from build123d import *

# Parameters (mm, degrees)
BOSS_EXTRUDE1_DEPTH          = 2.65684
CUT_EXTRUDE1_DEPTH           = 3.65684
SKETCH3_R                    = 16.891
CUT_EXTRUDE2_DEPTH           = 3.65684
F_10_0_1935_DIAMETER_HOLE1_D = 4.9149


with BuildPart() as part:
    # Sketch1 → Boss-Extrude1 (new body)
    with BuildSketch(Plane(origin=(0, 0, 0), x_dir=(1, 0, 0), z_dir=(0, 1, 0))):
        Polygon((-711.2, 203.2), (-711.2, 0), (711.2, 0), (711.2, 203.2), (330.2, 812.8), (-330.2, 812.8), align=None)
    extrude(amount=BOSS_EXTRUDE1_DEPTH)

    # Sketch2 → Cut-Extrude1 (cut, through all)
    with BuildSketch(Plane(origin=(0, 2.65684, 0), x_dir=(1, 0, 0), z_dir=(0, 1, 0))):
        with BuildLine():
            Line((-63.5, 781.05), (63.5, 781.05))
            ThreePointArc((63.5, 781.05), (79.375, 765.175), (63.5, 749.3))
            Line((63.5, 749.3), (-63.5, 749.3))
            ThreePointArc((-63.5, 749.3), (-79.375, 765.175), (-63.5, 781.05))
        make_face()
        with BuildLine():
            Line((-647.7, 63.5), (-520.7, 63.5))
            ThreePointArc((-520.7, 63.5), (-504.825, 47.625), (-520.7, 31.75))
            Line((-520.7, 31.75), (-647.7, 31.75))
            ThreePointArc((-647.7, 31.75), (-663.575, 47.625), (-647.7, 63.5))
        make_face()
        with BuildLine():
            Line((520.7, 63.5), (647.7, 63.5))
            ThreePointArc((647.7, 63.5), (663.575, 47.625), (647.7, 31.75))
            Line((647.7, 31.75), (520.7, 31.75))
            ThreePointArc((520.7, 31.75), (504.825, 47.625), (520.7, 63.5))
        make_face()
    extrude(amount=-CUT_EXTRUDE1_DEPTH, mode=Mode.SUBTRACT)

    # Sketch3 → Cut-Extrude2 (cut, through all)
    with BuildSketch(Plane(origin=(0, 2.65684, 0), x_dir=(1, 0, 0), z_dir=(0, 1, 0))):
        with Locations((-469.9, 224.282)):
            Circle(SKETCH3_R)
        with Locations((-225.425, 669.586361505)):
            Circle(SKETCH3_R)
        with Locations((225.425, 669.586361505)):
            Circle(SKETCH3_R)
        with Locations((469.9, 224.282)):
            Circle(SKETCH3_R)
    extrude(amount=-CUT_EXTRUDE2_DEPTH, mode=Mode.SUBTRACT)

    # #10 (0.1935) Diameter Hole1 (through all)
    with Locations(Plane(origin=(0, 2.65684, 0), x_dir=(1, 0, 0), z_dir=(0, 1, 0))):
        with Locations((228.6, 25.4), (279.4, 25.4), (419.1, 76.2), (419.1, 127), (475.488, 76.2), (475.488, 127), (-475.488, 127), (-475.488, 76.2), (-419.1, 76.2), (-419.1, 127), (-279.4, 25.4), (-228.6, 25.4)):
            Hole(F_10_0_1935_DIAMETER_HOLE1_D / 2)


solid = part.part
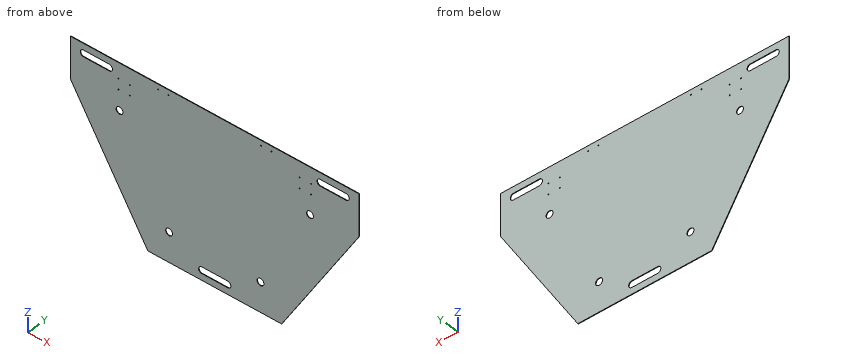
For this review, take the finished solid that the model builds, in its own axes (mm). Round coordinates to 2 decimals unless told otherwise and drop trailing zeros. Loops run counter-clockwise (first coordinate to the right, second up) from the corner with the lowest first, then second, coordinate; pieces in that order, holes last. Notation, with made-up numbers: (48, 48) - (102, 48) arc R26 cw to (102, 87) - close; hole circle Ø1 at (-16.75, 59.25). An arc over 180 degrees is marked (long way). Answer as CSV lines item,"result".
(1) Consider section D-D on z = -597. Give the boundary of the cut face in (x, y) (3 decimals).
Checked values:
outline,"(-465.075, 0) - (465.075, 0) - (465.075, 2.657) - (-465.075, 2.657) - close"
(2) Consider section A-A on x = -35. Give the boundary of the cut face in (y, z), then the cut area to 3 significant figures.
Checked values:
outline,"(0, -812.8) - (2.66, -812.8) - (2.66, -781.05) - (0, -781.05) - close; (0, -749.3) - (2.66, -749.3) - (2.66, 0) - (0, 0) - close"
area,"2,080 mm2"
(3) Consider section C-C on z = -256. Give the boundary of the cut face in (x, y).
Checked values:
outline,"(-678.2, 0) - (678.2, 0) - (678.2, 2.66) - (-678.2, 2.66) - close"
(4) Insertion check: P1, Ø1.3, axis at x = 598, y = 1.5, coming from the -Z side. The pin has a flat end and moves straight along its axis. Give the tip position at first contact, or say it passes through.
Checked values:
P1,"stops at z = -385.36"
(5) Consider section B-B on y = 2.1. Give the number of separate pieces and of enclosed holes in the cut face, then the cut area to 3 significant figures.
Checked values:
separate pieces,"1"
enclosed holes,"19"
area,"906,000 mm2"
(6) Wall thickness on line 1 (X direction, y = 1.5, z = -127); line 2 (X direction, y = 1.65, z = -25.4); line 3 (Z direction, x = -542.5, y = 2.55): over which ranges is each line inside the solid? List them lowest first.
Checked values:
line 1,"x = -711.2 to -477.95, -473.03 to -421.56, -416.64 to 416.64, 421.56 to 473.03, 477.95 to 711.2"
line 2,"x = -711.2 to -281.86, -276.94 to -231.06, -226.14 to 226.14, 231.06 to 276.94, 281.86 to 711.2"
line 3,"z = -473.12 to -63.5, -31.75 to 0"
